```python
from build123d import *

# Parameters (mm, degrees)
BOSS_EXTRUDE3_DEPTH = 150
SKETCH5_R           = 3.15
CUT_EXTRUDE1_DEPTH  = 10


with BuildPart() as part:
    # Sketch4 → Boss-Extrude3 (new body)
    with BuildSketch(Plane(origin=(0, 0, 0), x_dir=(1, 0, 0), z_dir=(0, 1, 0))):
        Polygon((8.948929172, -15.4), (17.840123318, 0), (8.920061659, 15.45), (-8.920061659, 15.45), (-17.811255804, 0.05), (-17.811255804, -22), (-63.584758496, -22), (-63.584758496, -15.35), (-23.584758496, -15.35), (-23.584758496, 0.05), (-11.806813005, 20.45), (11.806813005, 20.45), (23.61362601, 0), (13.279056191, -17.9), align=None)
    extrude(amount=-BOSS_EXTRUDE3_DEPTH)

    # Sketch5 → Cut-Extrude1 (cut)
    with BuildSketch(Plane(origin=(0, 0, 15.35), x_dir=(-1, 0, 0), z_dir=(0, 0, -1))):
        with Locations((43.584758496, -37.5)):
            Circle(SKETCH5_R)
        with Locations((43.584758496, -75)):
            Circle(SKETCH5_R)
        with Locations((43.584758496, -112.5)):
            Circle(SKETCH5_R)
    extrude(amount=-CUT_EXTRUDE1_DEPTH, mode=Mode.SUBTRACT)


solid = part.part
```
Check sheet for the modelled part. Datum: model origin and axes. Units: mm. A direction names the side the tool comes from. Coordinates: 2 decimals unless noted, no trailing zeros. Order: outer loops, then holes, each group sorted by start corner. A loop starts at its lowest first (then second) coordinate and runs counter-clockwise, first axis right, second up. Notation, with made-up numbers: M 29,7.25 L 67,7.25 A11 cw 67,24.25 Z; hole C 18,63 d9. An arc over 180 degrees is marked long. Write each question's results on one line, items separated by ' | '. Start each with the question number.
1. Go/stop test with flat-tipped pins: P1, Ø10, axis at y = -20, z = 7, coming from the -X side; P2, Ø12, axis at y = -22, z = -7.5, coming from the +X side; P3, Ø19.5, axis at x = -3, y = -39, coming from the +Z side. Record where each tip stops, or that it passes through.
2. Cross-section at C-C on y = -89. Record the cut outline in (x, z).
3. Access from +Z, -Z, +X, -X, +Y, -Y to the whole of each face (thin tool, end or side, straight path). Record for faces 1 (the face through (-23.585, -74, 8)), 2 (the face through (-17.811, -74, 11)), 3 (the face through (-45.038, -40.295, 18.628)), 4 (the face through (13.33, -73.95, 7.81)), 5 (the face through (-20, -150, 4)).
4. Cross-section at A-A on y = -112.5. Record the cut outline in (x, z).
5. Mould release check, pull along Y, two halves, no side actions. Record for faces 6 (the face through (18.52, -73.95, 8.82)), 7 (the face through (-45.278, -109.844, 18.628)), 8 (the face through (-20, 0, 4)): +Y half, -Y half, draft (parallel to the pull), parting line (faces both ways), or undercut.
6. Material ranges on probe 1 along X at (y, z) = (-37, 17); probe 2 along Z at (x, y) = (-2, -49); probe 3 along X at (y, z) = (-67.5, 17), recorded low to high.
7. Cross-section at B-B on z = 10. Record the cut outline in (x, y), and give its area (3 significant figures).
8. Cross-section at D-D on x = -49. Record the cut outline in (y, z).
Checks:
1) P1: stops at x = -23.58 | P2: stops at x = 22.75 | P3: stops at z = -8.82
2) outline: M -63.58,15.35 L -23.58,15.35 L -23.58,-0.05 L -11.81,-20.45 L 11.81,-20.45 L 23.61,0 L 13.28,17.9 L 8.95,15.4 L 17.84,0 L 8.92,-15.45 L -8.92,-15.45 L -17.81,-0.05 L -17.81,22 L -63.58,22 Z
3) face 1: -Z, -X, +Y, -Y | face 2: +Z, +Y, -Y | face 3: +Z, -Z | face 4: +Y, -Y | face 5: +Z, -Z, +X, -X, -Y
4) outline: M -63.58,15.35 L -46.73,15.35 L -46.73,22 L -63.58,22 Z; M -40.43,15.35 L -23.58,15.35 L -23.58,-0.05 L -11.81,-20.45 L 11.81,-20.45 L 23.61,0 L 13.28,17.9 L 8.95,15.4 L 17.84,0 L 8.92,-15.45 L -8.92,-15.45 L -17.81,-0.05 L -17.81,22 L -40.43,22 Z
5) face 6: draft | face 7: undercut | face 8: +Y half
6) probe 1: x = -63.58 to -46.69, -40.47 to -17.81, 11.72 to 13.8 | probe 2: z = -20.45 to -15.45 | probe 3: x = -63.58 to -17.81, 11.72 to 13.8
7) outline: M -23.58,-150 L -17.81,-150 L -17.81,0 L -23.58,0 Z; M 12.07,-150 L 17.84,-150 L 17.84,0 L 12.07,0 Z | area: 1,730 mm²
8) outline: M -150,15.35 L 0,15.35 L 0,22 L -150,22 Z
